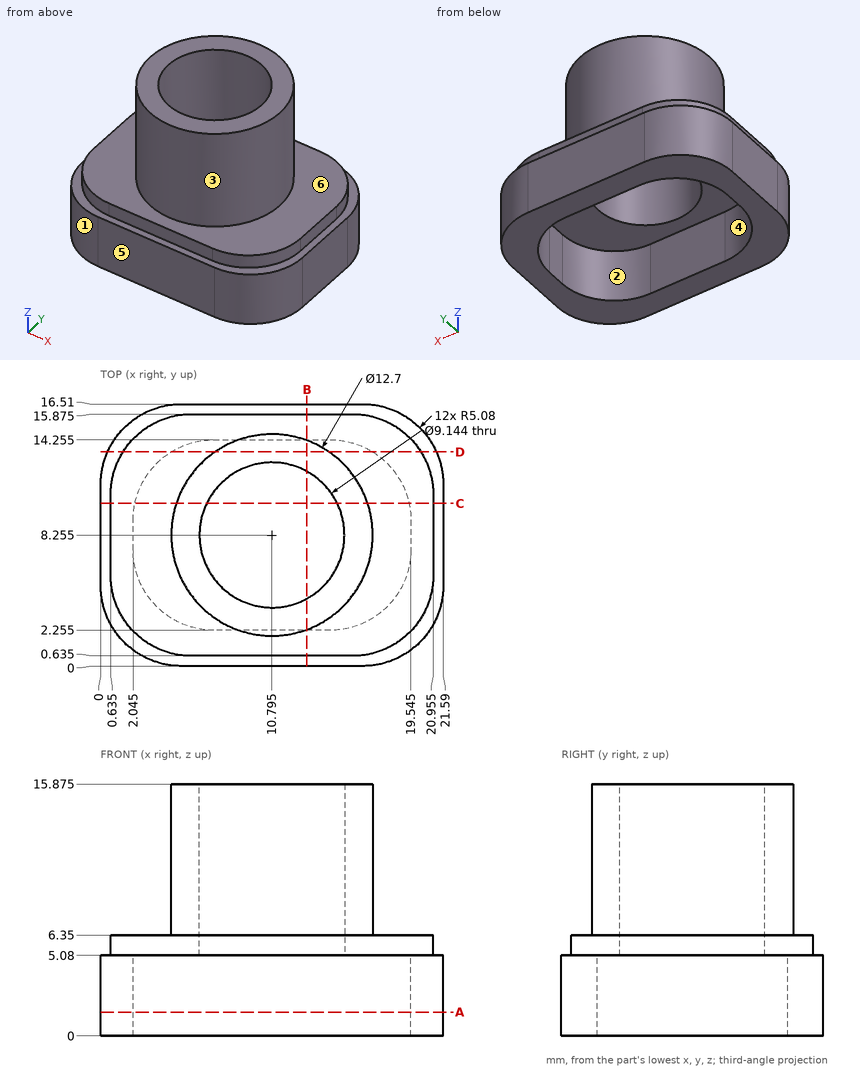
Could you check a few things on this drawing? It's one solid part, dimensions in mm from its lowest x, y, z. A direction names the side the tool comes from. Give positions to 0.01 mm unless a question says otherwise; leave off trailing zeros. Write each loop counter-clockwise with the first axis right and the second up, starting at its lowest first coordinate (ties: lowest second). Pieces come first, ordered by that corner, then holes. Notation, with made-up numbers: (77.5, -18) -> (115.5, -18) arc R20 cw to (115.5, 20) -> close; hole circle Ø8 at (-40, 50.5). An arc over 180 degrees is marked (long way). Answer as a JSON object with one key per item and string values.
Q1. Will these pins go through, and if not, where does the flat tip stop? pin 1 Ø1 at (x, z) = (6, 10.5) entering from +Y; pin 2 Ø3 at (x, z) = (3.5, 12.5) entering from +Y; pin 3 Ø5 at (x, z) = (11, 10) entering from -Y (3 decimals).
Taken from the geometry:
{"pin 1": "stops at y = 12.93", "pin 2": "stops at y = 10.85", "pin 3": "stops at y = 1.905"}
Q2. Suppose I cut it at C-C on y = 10.25. Write out the boundary of the cut face in (x, z) (3 decimals).
Taken from the geometry:
{"outline": "(0, 0) -> (2.16, 0) -> (2.16, 5.08) -> (6.681, 5.08) -> (6.681, 15.875) -> (4.767, 15.875) -> (4.767, 6.35) -> (0.635, 6.35) -> (0.635, 5.08) -> (0, 5.08) -> close; (14.909, 5.08) -> (19.43, 5.08) -> (19.43, 0) -> (21.59, 0) -> (21.59, 5.08) -> (20.955, 5.08) -> (20.955, 6.35) -> (16.823, 6.35) -> (16.823, 15.875) -> (14.909, 15.875) -> close"}
Q3. Which directions (+Z, -Z, +X, -X, +Y, -Y) give clear straight access to the entire face, cutting with the end or side of a thin tool? Please do the marked faces 4, 5 and 6.
Taken from the geometry:
{"face 4": "-Z", "face 5": "+Z, -Z, +X, -X, -Y", "face 6": "+Z"}
Q4. Please list where these lines run through material, in increasing order: L1, parallel to Y at x = 13.75, z = 1.75 (3 decimals); L2, parallel to X at y = 8, z = 3.75 (3 decimals); L3, parallel to Z at x = 18, y = 4.75.
Taken from the geometry:
{"L1": "y = 0 to 2.255, 14.255 to 16.51", "L2": "x = 0 to 2.045, 19.545 to 21.59", "L3": "z = 5.08 to 6.35"}
Q5. We'd pull the mould along Y, two halves only. Please class the marked faces 1, 2 and 3: released by +Y, released by -Y, zero draft, split by the parting line, or undercut.
Taken from the geometry:
{"face 1": "released by -Y", "face 2": "undercut", "face 3": "split by the parting line"}
Q6. Suppose I cut it at B-B on x = 13. Write out the boundary of the cut face in (y, z) (3 decimals), then the cut area to 3 significant figures.
Taken from the geometry:
{"outline": "(0, 0) -> (2.255, 0) -> (2.255, 5.08) -> (4.25, 5.08) -> (4.25, 15.875) -> (2.3, 15.875) -> (2.3, 6.35) -> (0.635, 6.35) -> (0.635, 5.08) -> (0, 5.08) -> close; (12.26, 5.08) -> (14.255, 5.08) -> (14.255, 0) -> (16.51, 0) -> (16.51, 5.08) -> (15.875, 5.08) -> (15.875, 6.35) -> (14.21, 6.35) -> (14.21, 15.875) -> (12.26, 15.875) -> close", "area": "69.2 mm²"}
Q7. Suppose I cut it at A-A on z = 1.5. Write out the boundary of the cut face in (x, y) (3 decimals), then the cut area to 3 significant figures.
Taken from the geometry:
{"outline": "(0, 5.08) arc R5.08 ccw to (5.08, 0) -> (16.51, 0) arc R5.08 ccw to (21.59, 5.08) -> (21.59, 11.43) arc R5.08 ccw to (16.51, 16.51) -> (5.08, 16.51) arc R5.08 ccw to (0, 11.43) -> close; hole (2.045, 7.335) arc R5.08 ccw to (7.125, 2.255) -> (14.465, 2.255) arc R5.08 ccw to (19.545, 7.335) -> (19.545, 9.175) arc R5.08 ccw to (14.465, 14.255) -> (7.125, 14.255) arc R5.08 ccw to (2.045, 9.175) -> close", "area": "146 mm²"}
Q8. Suppose I cut it at D-D on y = 13.5. Write out the boundary of the cut face in (x, z) (3 decimals).
Taken from the geometry:
{"outline": "(0.441, 0) -> (4.46, 0) -> (4.46, 5.08) -> (17.13, 5.08) -> (17.13, 0) -> (21.149, 0) -> (21.149, 5.08) -> (20.175, 5.08) -> (20.175, 6.35) -> (14.374, 6.35) -> (14.374, 15.875) -> (7.216, 15.875) -> (7.216, 6.35) -> (1.415, 6.35) -> (1.415, 5.08) -> (0.441, 5.08) -> close"}
